Autodesk Fusion 360 part; units mm, degrees
sketch "Sketch3" plane through (0, 0, 0) normal (0, 0, 1) x (1, 0, 0)
  line L0 (0, 0) -> (32, 0) construction
  line L1 (0, 0) -> (0, 48) construction
  line L2 (0, 0) -> (-32, 0) construction
  line L3 (32, 0) -> (32, -45)
  line L4 (-32, 0) -> (-32, -45)
  circle A0 centre (0, 0) radius 24.5 construction
  circle A1 centre (0, 0) radius 30.5 construction
  line L5 (0, 30.5) -> (-1.5, 30.5)
  line L6 (-32, 0) -> (-32, 0)
  arc A2 (-1.5, 30.5) -> (-32, 0) centre (-1.5, 0) ccw
  line L7 (32, 0) -> (32, 0)
  arc A3 (32, 0) -> (1.5, 30.5) centre (1.5, 0) ccw
  line L8 (0, 30.5) -> (1.5, 30.5)
  dimension "d22" = 32
  dimension "d23" = 45
  dimension "d24" = 45
  dimension "d25" = 49
  dimension "d26" = 6
  dimension "d27" = 30.5
sketch "Sketch4" plane through (0, 0, 0) normal (1, 0, 0) x (0, 0, -1)
  circle A0 centre (0, 30.5) radius 5
  point P0 (0, 30.5)
  dimension "d28" = 10
sweep "Sweep2" add profiles "Sketch4" path "Sketch3" along L3 A3 L8 L5 A2 L4 section 1
chamfer "Chamfer2" distance 1.5 angle 45 2 edges at (-33.8081, -45, 4.6616) (30.1919, -45, 4.6616)
thread "Thread3"
thread "Thread4"
equation "d22 = ( 64 / 2 ) * 1 mm"
For this review, take the finished solid that the model builds, in its own axes (mm). A direction names the side the tool comes from. Coordinates: 2 decimals unless noted, no trailing zeros. Loops run counter-clockwise (first coordinate to the right, second up) from the corner with the lowest first, then second, coordinate; pieces in that order, holes last.
1. Add section A-A, the plane z = 0. Give the boundary of the cut face in (x, y).
2. For line 1 (X direction, y = -13.5, z = -2); line 2 (X direction, y = -32.5, z = -1); line 3 (Y direction, x = 21, z = 1), list the stretches that pass through material, from the lowest coordinate up.
3. For faces 1 (the cylindrical face through (0.02, 25.62, 1.08)), 2 (the flat face through (-32, -45, 0)), 3 (the cylindrical face through (-27.12, -21.45, 1.08)), list the 3-axis set-ups (+Z, -Z, +X, -X, +Y, -Y) from which the entire face can be reached by the end or side of a thin tool; tool diameter is ignored.
4. Add section B-B, the plane y = -36.5. Give the boundary of the cut face in (x, z), then the cut area to 3 significant figures.
5. Insertion check: P1, Ø2, axis at y = 22.5, z = 1.5, coming from the +X side; P2, Ø2, axis at y = -19, z = -1.5, coming from the -X side; P3, Ø3, axis at y = 4, z = 2.5, coming from the -X side. Each pin has a flat end and moves straight along its axis. Give the tip position at first contact, or say it passes through.
6. Add section C-C, the plane x = 0.5. Give the boundary of the cut face in (y, z), then the cut area to 3 significant figures.
Result:
1. outline: (-37, -43.5) - (-35.5, -45) - (-28.5, -45) - (-27, -43.5) - (-27, 0) arc R25.5 cw to (-1.5, 25.5) - (1.5, 25.5) arc R25.5 cw to (27, 0) - (27, -43.5) - (28.5, -45) - (35.5, -45) - (37, -43.5) - (37, 0) arc R35.5 ccw to (1.5, 35.5) - (-1.5, 35.5) arc R35.5 ccw to (-37, 0) - close
2. line 1: x = -36.58 to -27.42, 27.42 to 36.58
2. line 2: x = -36.9 to -27.1, 27.1 to 36.9
2. line 3: y = 16.59 to 29.54
3. face 1: none
3. face 2: +Z, -Z, +X, -X, -Y
3. face 3: -Y
4. outline: circle Ø10 at (-32, 0); circle Ø10 at (32, 0)
4. area: 157 mm2
5. P1: stops at x = 29.53
5. P2: stops at x = -36.97
5. P3: stops at x = -36.71
6. outline: circle Ø10 at (30.5, 0)
6. area: 78.5 mm2
